Read the model definition and answer for the solid it produces. Units are mm, in the model's axes. A direction names the side the tool comes from. Give positions to 0.01 mm unless a question says otherwise; leave off trailing zeros. Order: outer loops, then holes, each group sorted by start corner. A loop starts at its lowest first (then second) coordinate and runs counter-clockwise, first axis right, second up. Notation, with made-up numbers: (-13, 5.25) - (16, 5.25) arc R11 ccw to (16, 13.25) - close; hole circle Ø6 at (-9, 6.5). An arc over 180 degrees is marked (long way). Return JSON: item names as keys, results as strings.
```python
from build123d import *

# Parameters (mm, degrees)
F0_W     = 10
F0_H     = 3
F1_DEPTH = 10
F2_R     = 2.15
F3_DEPTH = 6
F5_DEPTH = 2.5
F6_R     = 3.65
F7_DEPTH = 3
F9_DEPTH = 3


with BuildPart() as f1:
    # F0 (on Right) → F1 (new body)
    with BuildSketch(Plane.YZ):
        Polygon((-10, -3.0702352835), (10, -3.0702352835), (10, 2.9297647165), (-10, 2.9297647165), (-10, 1.4297647165), (0, 1.4297647165), (0, -1.5702352835), (-10, -1.5702352835), align=None)
        with Locations((-5, -0.0702352835)):
            Rectangle(F0_W, F0_H)
    extrude(amount=F1_DEPTH)

    # F2 (on face) → F3 (cut, through all)
    with BuildSketch(Plane.XY.offset(2.9297647165)):
        with Locations((5, -5)):
            Circle(F2_R)
        with BuildLine():
            ThreePointArc((6.75, 5), (6.6167891819, 5.6696960066), (6.2374368671, 6.2374368671))
            Line((6.2374368671, 6.2374368671), (3.7625631329, 3.7625631329))
            ThreePointArc((3.7625631329, 3.7625631329), (5.6696960066, 3.3832108181), (6.75, 5))
        make_face()
        with BuildLine():
            Line((3.7625631329, 3.7625631329), (6.2374368671, 6.2374368671))
            ThreePointArc((6.2374368671, 6.2374368671), (3.7625631329, 6.2374368671), (3.7625631329, 3.7625631329))
        make_face()
    extrude(amount=-F3_DEPTH, mode=Mode.SUBTRACT)

    # F4 (on face) → F5 (cut)
    with BuildSketch(Plane(origin=(0, 0, -3.0702352835), x_dir=(1, 0, 0), z_dir=(0, 0, -1))):
        Polygon((1.7668389044, -5.0016318656), (3.3848326892, -7.8008155761), (6.6179937849, -7.7991837106), (8.2331610956, -4.9983681344), (6.6151673108, -2.1991844239), (3.3820062151, -2.2008162894), align=None)
    extrude(amount=-F5_DEPTH, mode=Mode.SUBTRACT)

    # F6 (on face) → F7 (cut)
    with BuildSketch(Plane.XY.offset(2.9297647165)):
        with Locations((5, -5)):
            Circle(F6_R)
    extrude(amount=-F7_DEPTH, mode=Mode.SUBTRACT)

    # F8 (on face) → F9 (cut)
    with BuildSketch(Plane.XY.offset(2.9297647165)):
        with BuildLine():
            Line((0, -5.6770486943), (0, -10))
            Line((0, -10), (10, -10))
            Line((10, -10), (10, -5.6770486943))
            ThreePointArc((10, -5.6770486943), (5, -1.3859687615), (0, -5.6770486943))
        make_face()
    extrude(amount=-F9_DEPTH, mode=Mode.SUBTRACT)


solid = f1.part
```
Q1. Consider L1, parallel to Y at x = 5, z = -1.1; L2, parallel to Z at x = 2.5, y = -7.5; L3, parallel to Y at x = 3.5, z = 2.7. Determine where each line is inside the solid, lowest interval first.
Values:
{"L1": "y = -10 to -7.15, -2.85 to 2.2, 7.8 to 10", "L2": "z = -3.07 to -0.07", "L3": "y = -1.61 to 4.1, 5.9 to 10"}
Q2. A cutting plane is placed at D-D (z = -2.35). Write down the section's boundary in (x, y), and give its area (3 significant figures).
Values:
{"outline": "(0, -10) - (10, -10) - (10, 10) - (0, 10) - close; hole (1.77, 5) - (3.38, 2.2) - (6.62, 2.2) - (8.23, 5) - (6.62, 7.8) - (3.38, 7.8) - close; hole circle Ø4.3 at (5, -5)", "area": "158 mm²"}
Q3. A cutting plane is placed at B-B (x = 5). Write down the section's boundary in (y, z).
Values:
{"outline": "(-10, -3.07) - (-7.15, -3.07) - (-7.15, -0.07) - (-10, -0.07) - close; (-2.85, -3.07) - (2.2, -3.07) - (2.2, -0.57) - (3.25, -0.57) - (3.25, 2.93) - (-1.35, 2.93) - (-1.35, -0.07) - (-2.85, -0.07) - close; (6.75, -0.57) - (7.8, -0.57) - (7.8, -3.07) - (10, -3.07) - (10, 2.93) - (6.75, 2.93) - close"}
Q4. For faces 1 (the flat face through (2.586, 3.582, -1.838)), 2 (the cylindrical face through (5.01, -1.35, 1.45)), 3 (the flat face through (5, 0, -3.07)), determine the directions among +Z, -Z, +X, -X, +Y, -Y from which every point of the face is accessible in a straight line to the end or side of a thin tool.
Values:
{"face 1": "-Z", "face 2": "+Z, -Y", "face 3": "-Z, +X, -X, +Y, -Y"}
Q5. Given pin 1 (5 mm diameter, centred on x = 5, y = -5, fed in from +Z), flat-ended and moving along its own axis, determine where the tip first touches the part or whether it passes through.
Values:
{"pin 1": "stops at z = -0.07"}
Q6. Determine the mould class of faces 4 (the cylindrical face through (1.39, -2.9, 1.45)), 5 (the flat face through (0, 0, 0)), 6 (the cylindrical face through (3.294, -6.308, -1.549)) for opening direction Y: released by +Y, released by -Y, zero draft, split by the parting line, or undercut.
Values:
{"face 4": "released by -Y", "face 5": "zero draft", "face 6": "undercut"}
Q7. A cutting plane is placed at A-A (z = 2.5). Write down the section's boundary in (x, y).
Values:
{"outline": "(0, -5.68) arc R5.06 cw to (4.05, -1.48) arc R3.65 cw to (5.95, -1.48) arc R5.06 cw to (10, -5.68) - (10, 10) - (0, 10) - close; hole circle Ø3.5 at (5, 5)"}
Q8. A cutting plane is placed at C-C (y = 5.5). Write down the section's boundary in (x, z).
Values:
{"outline": "(0, -3.07) - (2.05, -3.07) - (2.05, -0.57) - (3.32, -0.57) - (3.32, 2.93) - (0, 2.93) - close; (6.68, -0.57) - (7.94, -0.57) - (7.94, -3.07) - (10, -3.07) - (10, 2.93) - (6.68, 2.93) - close"}
